from build123d import *

# Parameters (mm, degrees)
BOSS_EXTRUDE1_DEPTH = 4
FILLET1_R           = 5
FILLET2_R           = 20
SKETCH3_R           = 2
CUT_EXTRUDE1_DEPTH  = 5
SKETCH4_R           = 2
CUT_EXTRUDE2_DEPTH  = 10
SKETCH5_W           = 262
SKETCH5_H           = 8
BOSS_EXTRUDE2_DEPTH = 4


with BuildPart() as part:
    # Sketch1 → Boss-Extrude1 (new body)
    with BuildSketch(Plane(origin=(0, 0, 0), x_dir=(1, 0, 0), z_dir=(0, 1, 0))):
        Polygon((128, 112.5), (148, 112.5), (148, -112.5), (128, -112.5), (128, -80.5), (-128, -80.5), (-128, -112.5), (-148, -112.5), (-148, 112.5), (-128, 112.5), (-128, 80.5), (128, 80.5), align=None)
    extrude(amount=BOSS_EXTRUDE1_DEPTH)

    # Fillet1
    fillet1_edges = [part.edges().sort_by_distance(p)[0] for p in [
        (148, 2, 112.5),
        (128, 2, 112.5),
        (-128, 2, 112.5),
        (-148, 2, 112.5),
        (-148, 2, -112.5),
        (-128, 2, -112.5),
        (128, 2, -112.5),
        (148, 2, -112.5),
    ]]
    fillet(fillet1_edges, radius=FILLET1_R)

    # Fillet2
    fillet2_edges = [part.edges().sort_by_distance(p)[0] for p in [
        (128, 2, 80.5),
        (-128, 2, 80.5),
        (-128, 2, -80.5),
        (128, 2, -80.5),
    ]]
    fillet(fillet2_edges, radius=FILLET2_R)

    # Sketch3 → Cut-Extrude1 (cut)
    with BuildSketch(Plane(origin=(0, 4, 0), x_dir=(1, 0, 0), z_dir=(0, 1, 0))):
        with Locations(Location((-140.5, 102.5, 0), (0, 0, 270))):
            Circle(SKETCH3_R)
        with Locations(Location((140.5, 102.5, 0), (0, 0, 270))):
            Circle(SKETCH3_R)
        with Locations(Location((140.5, -102.5, 0), (0, 0, 270))):
            Circle(SKETCH3_R)
        with Locations(Location((-140.5, -102.5, 0), (0, 0, 270))):
            Circle(SKETCH3_R)
    extrude(amount=-CUT_EXTRUDE1_DEPTH, mode=Mode.SUBTRACT)

    # Sketch4 → Cut-Extrude2 (cut)
    with BuildSketch(Plane(origin=(0, 4, 0), x_dir=(1, 0, 0), z_dir=(0, 1, 0))):
        with Locations(Location((-136, 66.5, 0), (0, 0, 270))):
            Circle(SKETCH4_R)
        with Locations(Location((-136, 15.5, 0), (0, 0, 270))):
            Circle(SKETCH4_R)
        with Locations(Location((-106, 15.5, 0), (0, 0, 270))):
            Circle(SKETCH4_R)
        with Locations(Location((-106, 66.5, 0), (0, 0, 270))):
            Circle(SKETCH4_R)
        with Locations(Location((-90.8, 75.5, 0), (0, 0, 270))):
            Circle(SKETCH4_R)
        with Locations(Location((-90.8, 49.5, 0), (0, 0, 270))):
            Circle(SKETCH4_R)
        with Locations(Location((-33.3, 75.5, 0), (0, 0, 270))):
            Circle(SKETCH4_R)
        with Locations(Location((-33.3, 49.5, 0), (0, 0, 270))):
            Circle(SKETCH4_R)
        with Locations(Location((3, 71.5, 0), (0, 0, 270))):
            Circle(SKETCH4_R)
        with Locations(Location((61, 71.5, 0), (0, 0, 270))):
            Circle(SKETCH4_R)
        with Locations(Location((61, 22.5, 0), (0, 0, 270))):
            Circle(SKETCH4_R)
        with Locations(Location((3, 22.5, 0), (0, 0, 270))):
            Circle(SKETCH4_R)
        with Locations(Location((66, 14.5, 0), (0, 0, 270))):
            Circle(SKETCH4_R)
        with Locations(Location((123, 14.5, 0), (0, 0, 270))):
            Circle(SKETCH4_R)
        with Locations(Location((123, -50.5, 0), (0, 0, 270))):
            Circle(SKETCH4_R)
        with Locations(Location((66, -50.5, 0), (0, 0, 270))):
            Circle(SKETCH4_R)
        with Locations(Location((94.5, 43.5, 0), (0, 0, 270))):
            Circle(SKETCH4_R)
        with Locations(Location((94.5, -70.5, 0), (0, 0, 270))):
            Circle(SKETCH4_R)
        with Locations(Location((-128, -7.5, 0), (0, 0, 270))):
            Circle(SKETCH4_R)
        with Locations(Location((-128, -65.5, 0), (0, 0, 270))):
            Circle(SKETCH4_R)
        with Locations(Location((-61, -64.5, 0), (0, 0, 270))):
            Circle(SKETCH4_R)
        with Locations(Location((-61, -3.5, 0), (0, 0, 270))):
            Circle(SKETCH4_R)
        with Locations(Location((-38.5, -3.5, 0), (0, 0, 270))):
            Circle(SKETCH4_R)
    extrude(amount=-CUT_EXTRUDE2_DEPTH, mode=Mode.SUBTRACT)

    # Sketch5 → Boss-Extrude2 (add)
    with BuildSketch(Plane.XZ):
        with Locations((0, 40.5)):
            Rectangle(SKETCH5_W, SKETCH5_H)
        with Locations((0, -5.5)):
            Rectangle(SKETCH5_W, SKETCH5_H)
        with Locations((0, -57.5)):
            Rectangle(SKETCH5_W, SKETCH5_H)
    extrude(amount=BOSS_EXTRUDE2_DEPTH)


solid = part.part
Can you work these out from the model? Positions are in its coordinate system, mm. A direction names the side the tool comes from. Round coordinates to 2 decimals unless told otherwise and drop trailing zeros. Loops run counter-clockwise (first coordinate to the right, second up) from the corner with the lowest first, then second, coordinate; pieces in that order, holes last. Notation, with made-up numbers: (78, -34) - (132, -34) arc R23 ccw to (132, -23) - close; hole circle Ø7 at (77.25, -15.75). An arc over 180 degrees is marked (long way). Answer in a Markdown table with one row per item. Add a question column.
Q1. Which directions (+Z, -Z, +X, -X, +Y, -Y) give clear straight access to the entire face, cutting with the end or side of a thin tool? Please do faces 3 (the flat face through (2, 4, -2)), 4 (the cylindrical face through (122.297, 2.028, -86.514)), 5 (the cylindrical face through (122.297, 2.028, 86.514)).
Q2. We'd pull the mould along X, two halves only. Please class faces 1 (the flat face through (-2, -4, -5)), 2 (the cylindrical face through (-121.986, 2.028, -86.203)): pulls with the +X half, pulls with the -X half, needs draft (parallel to the pull), parting line crosses it, or undercut.
Q3. I want a section at B-B on x = 89.5. List the corners of the cut face in (y, z) for me, and give its area (3 significant figures).
Q4. I need wall thicknesses on L1, parallel to Z at x = 140.5, y = 2.85; L2, parallel to Z at x = 121.5, y = -1.75; L3, parallel to X at y = 0.8, z = -102.5. Which ranges of each line are inside material? Lowest first, please.
Q5. For pin 1 Ø8 at (x, z) = (60.5, 61.5) entering from -Y; pin 2 Ø2.5 at (x, z) = (-136, -15.5) entering from -Y; pin 3 Ø1.2 at (x, y) = (63, -1.5) entering from +Z; pin 4 Ø3 at (y, z) = (-2.5, 41.5) entering from +X, each with a flat end and sliding along its axis, tell me the tip position at first contact or that it passes through.
Q6. I want a section at A-A on y = -1.5. List the corners of the cut face in (x, z) for me.
Q7. I want a section at C-C on z = 26.5. List the corners of the cut face in (x, y) for me, and give its area (3 significant figures).
A:
| question | item | result |
|---|---|---|
| 1 | face 3 | +Z, -Z, +X, -X, +Y |
| 1 | face 4 | -Z, +Y, -Y |
| 1 | face 5 | +Z, +Y, -Y |
| 2 | face 1 | needs draft |
| 2 | face 2 | undercut |
| 3 | outline | (-4, -61.5) - (0, -61.5) - (0, -80.5) - (4, -80.5) - (4, 80.5) - (0, 80.5) - (0, 44.5) - (-4, 44.5) - (-4, 36.5) - (0, 36.5) - (0, -1.5) - (-4, -1.5) - (-4, -9.5) - (0, -9.5) - (0, -53.5) - (-4, -53.5) - close |
| 3 | area | 740 mm^2 |
| 4 | L1 | -112.5 to -104.5, -100.5 to 100.5, 104.5 to 112.5 |
| 4 | L2 | -61.5 to -53.5, -9.5 to -1.5, 36.5 to 44.5 |
| 4 | L3 | -148 to -142.5, -138.5 to -128, 128 to 138.5, 142.5 to 148 |
| 5 | pin 1 | y = 0 |
| 5 | pin 2 | through |
| 5 | pin 3 | z = 44.5 |
| 5 | pin 4 | x = 131 |
| 6 | outline | (-131, -61.5) - (131, -61.5) - (131, -53.5) - (-131, -53.5) - close; (-131, -9.5) - (131, -9.5) - (131, -1.5) - (-131, -1.5) - close; (-131, 36.5) - (131, 36.5) - (131, 44.5) - (-131, 44.5) - close |
| 7 | outline | (-148, 0) - (148, 0) - (148, 4) - (-148, 4) - close |
| 7 | area | 1,180 mm^2 |
